Geometry check sheet. Reference: drawing and pictorial views, mm from the part's lowest x, y, z. Give positions to 0.01 mm unless a question says otherwise; leave off trailing zeros. Loops run counter-clockwise (first coordinate to the right, second up) from the corner with the lowest first, then second, coordinate; pieces in that order, holes last. Notation, with made-up numbers: (43, -34.75) - (49, -34.75) arc R16 ccw to (49, -16.75) - close; hole circle Ø5 at (45, 1.25). An arc over 180 degrees is marked (long way). One line per question, with ' | ' between items. Start each with the question number.
1. Section check A-A, the plane z = 2.5. Enter the section's corners in (x, y) (1 decimal), then the cut area to 3 significant figures.
2. Mould release check, pull along Y, two halves, no side actions. Record for the marked faces 1, 2, 3 and 4: +Y half, -Y half, draft (parallel to the pull), parting line (faces both ways), or undercut.
3. Depth check by flat-ended pin: pin 1 Ø4 at (y, z) = (9, 4.5) entering from -X; pin 2 Ø4 at (y, z) = (5, 2.5) entering from +X; pin 3 Ø1 at (y, z) = (11, 5.5) entering from -X. Enter the tip coordinate at first touch or a pass-through.
4. Thickness scan on line 1 along X through (y, z) = (9.75, 4.5) (1 decimal); line 2 along Y through (x, z) = (11.5, 3) (1 decimal); line 3 along Y through (x, z) = (11.75, 6.5). Record the ranges inside material, lowest first. Write a range as from..to.
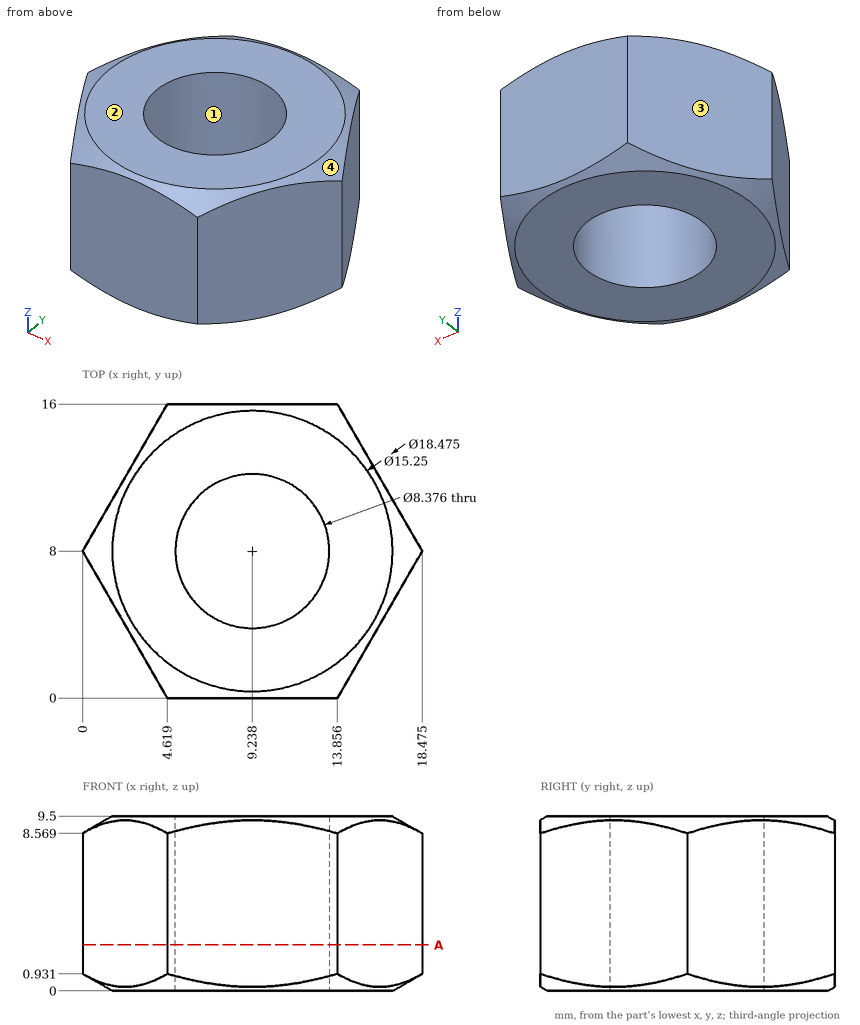
Results list:
1) outline: (0, 8) - (4.6, 0) - (13.9, 0) - (18.5, 8) - (13.9, 16) - (4.6, 16) - close; hole circle Ø8.4 at (9.2, 8) | area: 167 mm²
2) face 1: undercut | face 2: draft | face 3: +Y half | face 4: parting line
3) pin 1: x = 0 | pin 2: x = 17.9 | pin 3: x = 1.44
4) line 1: 1..5.4, 13..17.5 | line 2: 0..4.5, 11.5..16 | line 3: 0..4.65, 11.35..16
